Part model, mm, in its own coordinate system. Round coordinates to 2 decimals unless told otherwise and drop trailing zeros. Loops run counter-clockwise (first coordinate to the right, second up) from the corner with the lowest first, then second, coordinate; pieces in that order, holes last. Notation, with made-up numbers: (-36.75, -23) - (-0.75, -23) arc R12 ccw to (-0.75, -5) - close; hole circle Ø9 at (-18.75, -35). An arc over 180 degrees is marked (long way). Write each question's results on one line, items separated by ' | '. Start each with the question number.
(1) Flat gauge pin, fed straight in: P1, Ø6.5, axis at x = 86.16, z = -15.44, coming from the +Y side. Where does the tip first touch, or does it go through?
(2) Cut at B-B, the plane y = 10.75. List the corners of the cut face in (x, z).
(3) Cut at A-A, the plane z = -50.8. List the corners of the cut face in (x, y).
(4) Drill centre lines: L1, parallel to X at y = 1, z = -88.5; L2, parallel to Z at x = 12.7, y = 6; L3, parallel to X at y = 6.75, z = -47.5. Where is each one in solid material? Low to high.
(5) Cut at C-C, the plane x = 12.7. List the corners of the cut face in (y, z).
(6) Mould opens along X. For faces 1 (the face through (16.13, 6.26, -20.65)), 2 (the face through (81.148, 6.261, -87.732)), 3 (the face through (101.6, 6, -50)), 4 (the face through (50, 6, -101.6)) say: released by +X, released by -X, zero draft, split by the parting line, or undercut.
from build123d import *

# Parameters (mm, degrees)
SKETCH1_W               = 101.6
SKETCH1_H               = 101.6
BOSS_EXTRUDE1_DEPTH     = 12.7
M10_CLEARANCE_HOLE1_D   = 10.5
F_1_2_13_TAPPED_HOLE1_D = 10.71626


with BuildPart() as part:
    # Sketch1 → Boss-Extrude1 (new body)
    with BuildSketch(Plane(origin=(0, 0, 0), x_dir=(1, 0, 0), z_dir=(0, 1, 0))):
        with Locations((50.8, 50.8)):
            Rectangle(SKETCH1_W, SKETCH1_H)
    extrude(amount=BOSS_EXTRUDE1_DEPTH)

    # M10 Clearance Hole1 (through all)
    with Locations(Plane(origin=(0, 12.7, 0), x_dir=(1, 0, 0), z_dir=(0, 1, 0))):
        with Locations((86.155339059, 86.155339059), (86.155339059, 15.444660941), (15.444660941, 86.155339059), (15.444660941, 15.444660941)):
            Hole(M10_CLEARANCE_HOLE1_D / 2)

    # 1/2-13 Tapped Hole1 (through all)
    with Locations(Plane(origin=(0, 12.7, 0), x_dir=(1, 0, 0), z_dir=(0, 1, 0))):
        with Locations((88.9, 50.8), (12.7, 50.8)):
            Hole(F_1_2_13_TAPPED_HOLE1_D / 2)


solid = part.part
A:
1) P1: through
2) outline: (0, -101.6) - (101.6, -101.6) - (101.6, 0) - (0, 0) - close; hole circle Ø10.72 at (12.7, -50.8); hole circle Ø10.5 at (15.44, -86.16); hole circle Ø10.5 at (15.44, -15.44); hole circle Ø10.5 at (86.16, -86.16); hole circle Ø10.5 at (86.16, -15.44); hole circle Ø10.72 at (88.9, -50.8)
3) outline: (0, 0) - (7.34, 0) - (7.34, 12.7) - (0, 12.7) - close; (18.06, 0) - (83.54, 0) - (83.54, 12.7) - (18.06, 12.7) - close; (94.26, 0) - (101.6, 0) - (101.6, 12.7) - (94.26, 12.7) - close
4) L1: 0 to 10.75, 20.14 to 81.46, 90.85 to 101.6 | L2: -101.6 to -90.63, -81.68 to -56.16, -45.44 to -19.92, -10.97 to 0 | L3: 0 to 8.48, 16.92 to 84.68, 93.12 to 101.6
5) outline: (0, -101.6) - (12.7, -101.6) - (12.7, -90.63) - (0, -90.63) - close; (0, -81.68) - (12.7, -81.68) - (12.7, -56.16) - (0, -56.16) - close; (0, -45.44) - (12.7, -45.44) - (12.7, -19.92) - (0, -19.92) - close; (0, -10.97) - (12.7, -10.97) - (12.7, 0) - (0, 0) - close
6) face 1: undercut | face 2: undercut | face 3: released by +X | face 4: zero draft
